Build history of the part. All positions in model axes, mm. A direction names the side the tool comes from. Give positions to 0.01 mm unless a question says otherwise; leave off trailing zeros. Order: outer loops, then holes, each group sorted by start corner. A loop starts at its lowest first (then second) coordinate and runs counter-clockwise, first axis right, second up. Notation, with made-up numbers: (2.5, 6.5) -> (56.5, 6.5) arc R31 cw to (56.5, 43.5) -> close; hole circle Ø2 at (27, 12). An arc over 180 degrees is marked (long way). Write item = value, one per line. Start each with the question number.
from build123d import *

# Parameters (mm, degrees)
SKETCH_1_W               = 74
SKETCH_1_H               = 52
EXTRUDE_1_DEPTH          = 2
CUT_EXTRUDE_2_DEPTH      = 10
SKETCH_3_W               = 2
SKETCH_3_H               = 8
EXTRUDE_3_DEPTH          = 7.5
FILLET_1_R               = 2
FILLET_1_OF_MIRROR_3_R   = 2
MIRROR_4_DEPTH           = 2
EXTRUDE_4_DEPTH          = 2
FILLET_3_R               = 1
FILLET_4_R               = 2
SKETCH_4_R               = 1.5
CUT_EXTRUDE_3_DEPTH      = 6
SKETCH_5_R               = 1
CUT_EXTRUDE_5_DEPTH      = 6
MIRROR_6_COPY_1_SKETCH_R = 1
MIRROR_6_COPY_1_DEPTH    = 6
SKETCH_6_R               = 1
CUT_EXTRUDE_6_DEPTH      = 10
MIRROR_9_COPY_1_SKETCH_R = 1
MIRROR_9_COPY_1_DEPTH    = 10
FILLET_5_R               = 1
CUT_EXTRUDE_7_DEPTH      = 10
MIRROR_12_COPY_1_DEPTH   = 10


# Read off the part's stored shape, not the designer's step: 镜向4
with BuildPart() as part:
    # 草图1 → 凸台-拉伸1 (new body)
    with BuildSketch(Plane(origin=(0, 0, 0), x_dir=(0, 0, -1), z_dir=(1, 0, 0))):
        Rectangle(SKETCH_1_W, SKETCH_1_H)
    extrude(amount=EXTRUDE_1_DEPTH)

    # 草图2 → 切除-拉伸2 (cut)
    with BuildSketch(Plane(origin=(2, 0, 0), x_dir=(0, 0, -1), z_dir=(1, 0, 0))):
        Polygon((-7, 0), (-31, 26), (-37, 26), (-37, -26), (-31, -26), align=None)
        Polygon((17, 26), (-17, 26), (0, 7.583333333), align=None)
        Polygon((31, 26), (7, 0), (31, -26), (37, -26), (37, 26), align=None)
        Polygon((17, -26), (0, -7.583333333), (-17, -26), align=None)
    extrude(amount=-CUT_EXTRUDE_2_DEPTH, mode=Mode.SUBTRACT)

    # 草图3 → 凸台-拉伸3 (add)
    with BuildSketch(Plane(origin=(0, 26, 0), x_dir=(1, 0, 0), z_dir=(0, 1, 0))):
        with Locations((1, -24)):
            Rectangle(SKETCH_3_W, SKETCH_3_H)
    extrude_3 = extrude(amount=EXTRUDE_3_DEPTH)

    # 圆角1
    fillet_1_edges = [part.edges().sort_by_distance(p)[0] for p in [
        (1, 33.5, 28),
        (1, 33.5, 20),
    ]]
    fillet(fillet_1_edges, radius=FILLET_1_R)

    # 镜向3: 凸台-拉伸3 across plane
    add(extrude_3.mirror(Plane.XY))

    # 圆角1 of 镜向3
    fillet_1_of_mirror_3_edges = [part.edges().sort_by_distance(p)[0] for p in [
        (1, 33.5, -28),
        (1, 33.5, -20),
    ]]
    fillet(fillet_1_of_mirror_3_edges, radius=FILLET_1_OF_MIRROR_3_R)

    # 镜向4 outline → 镜向4 (add)
    with BuildSketch(Plane.YZ):
        with BuildLine():
            Line((-26, 20), (-26, 28))
            Line((-26, 28), (-31.5, 28))
            ThreePointArc((-31.5, 28), (-32.914213562, 27.414213562), (-33.5, 26))
            Line((-33.5, 26), (-33.5, 22))
            ThreePointArc((-33.5, 22), (-32.914213562, 20.585786438), (-31.5, 20))
            Line((-31.5, 20), (-26, 20))
        make_face()
        with BuildLine():
            Line((-26, -20), (-31.5, -20))
            ThreePointArc((-31.5, -20), (-32.914213562, -20.585786438), (-33.5, -22))
            Line((-33.5, -22), (-33.5, -26))
            ThreePointArc((-33.5, -26), (-32.914213562, -27.414213562), (-31.5, -28))
            Line((-31.5, -28), (-26, -28))
            Line((-26, -28), (-26, -20))
        make_face()
    extrude(amount=MIRROR_4_DEPTH)

    # 草图7 → 凸台-拉伸4 (add)
    with BuildSketch(Plane(origin=(2, 0, 0), x_dir=(0, 0, -1), z_dir=(1, 0, 0))):
        Polygon((-28, 26), (-33, 26), (-33, 21.44166802), (-19, 13), align=None)
        Polygon((19, 13), (28, 26), (33, 26), (33, 21.44166802), align=None)
        Polygon((28, -26), (33, -26), (33, -21.44166802), (19, -13), align=None)
        Polygon((-19, -13), (-28, -26), (-33, -26), (-33, -21.44166802), align=None)
    extrude(amount=-EXTRUDE_4_DEPTH)

    # 圆角3
    fillet_3_edges = [part.edges().sort_by_distance(p)[0] for p in [
        (1, 26, 33),
        (1, 21.44166802, 33),
        (1, 26, -33),
        (1, 21.44166802, -33),
        (1, -26, -33),
        (1, -21.44166802, -33),
        (1, -26, 33),
        (1, -21.44166802, 33),
    ]]
    fillet(fillet_3_edges, radius=FILLET_3_R)

    # 圆角4
    fillet_4_edges = [part.edges().sort_by_distance(p)[0] for p in [
        (1, 0, -7),
        (1, 26, -17),
        (1, 7.583333333, 0),
        (1, 26, 17),
        (1, -7.583333333, 0),
        (1, -26, -17),
        (1, -26, 17),
        (1, 0, 7),
    ]]
    fillet(fillet_4_edges, radius=FILLET_4_R)

    # 草图4 → 切除-拉伸3 (cut)
    with BuildSketch(Plane(origin=(2, 0, 0), x_dir=(0, 0, -1), z_dir=(1, 0, 0))):
        with Locations((0, -4.5)):
            Circle(SKETCH_4_R)
        with Locations((-4.5, 0)):
            Circle(SKETCH_4_R)
        with Locations((0, 4.5)):
            Circle(SKETCH_4_R)
        with Locations((4.5, 0)):
            Circle(SKETCH_4_R)
    extrude(amount=-CUT_EXTRUDE_3_DEPTH, mode=Mode.SUBTRACT)

    # 草图5 → 切除-拉伸5 (cut)
    with BuildSketch(Plane(origin=(2, 0, 0), x_dir=(0, 0, -1), z_dir=(1, 0, 0))):
        with Locations((-24, 30.5)):
            Circle(SKETCH_5_R)
        with BuildLine():
            ThreePointArc((-23, 30.5), (-24, 29.5), (-25, 30.5))
            Line((-25, 30.5), (-25, 23.5))
            ThreePointArc((-25, 23.5), (-24, 24.5), (-23, 23.5))
            Line((-23, 23.5), (-23, 30.5))
        make_face()
        with Locations((-24, 23.5)):
            Circle(SKETCH_5_R)
    cut_extrude_5 = extrude(amount=-CUT_EXTRUDE_5_DEPTH, mode=Mode.SUBTRACT)

    # 镜向5: 切除-拉伸5 across plane
    add(cut_extrude_5.mirror(Plane.XY), mode=Mode.SUBTRACT)

    # 镜向6: 切除-拉伸5 across plane
    add(cut_extrude_5.mirror(Plane.ZX), mode=Mode.SUBTRACT)

    # 镜向6 copy 1 sketch → 镜向6 copy 1 (cut)
    with BuildSketch(Plane(origin=(2, 0, 0), x_dir=(0, 0, 1), z_dir=(1, 0, 0))):
        with Locations((-24, 30.5)):
            Circle(MIRROR_6_COPY_1_SKETCH_R)
        with BuildLine():
            ThreePointArc((-23, 30.5), (-24, 29.5), (-25, 30.5))
            Line((-25, 30.5), (-25, 23.5))
            ThreePointArc((-25, 23.5), (-24, 24.5), (-23, 23.5))
            Line((-23, 23.5), (-23, 30.5))
        make_face()
        with Locations((-24, 23.5)):
            Circle(MIRROR_6_COPY_1_SKETCH_R)
    extrude(amount=-MIRROR_6_COPY_1_DEPTH, mode=Mode.SUBTRACT)

    # 草图6 → 切除-拉伸6 (cut)
    with BuildSketch(Plane(origin=(2, 0, 0), x_dir=(0, 0, -1), z_dir=(1, 0, 0))):
        with Locations((-20, 26)):
            Circle(SKETCH_6_R)
        with Locations((-28, 26)):
            Circle(SKETCH_6_R)
    cut_extrude_6 = extrude(amount=-CUT_EXTRUDE_6_DEPTH, mode=Mode.SUBTRACT)

    # 镜向8: 切除-拉伸6 across plane
    add(cut_extrude_6.mirror(Plane.ZX), mode=Mode.SUBTRACT)

    # 镜向9: 切除-拉伸6 across plane
    add(cut_extrude_6.mirror(Plane.XY), mode=Mode.SUBTRACT)

    # 镜向9 copy 1 sketch → 镜向9 copy 1 (cut)
    with BuildSketch(Plane(origin=(2, 0, 0), x_dir=(0, 0, 1), z_dir=(1, 0, 0))):
        with Locations((-20, 26)):
            Circle(MIRROR_9_COPY_1_SKETCH_R)
        with Locations((-28, 26)):
            Circle(MIRROR_9_COPY_1_SKETCH_R)
    extrude(amount=-MIRROR_9_COPY_1_DEPTH, mode=Mode.SUBTRACT)

    # 圆角5
    fillet_5_edges = [part.edges().sort_by_distance(p)[0] for p in [
        (1, 27, 20),
        (1, 27, 28),
        (1, 26, 19),
        (1, 26, 29),
        (1, -27, 28),
        (1, -27, 20),
        (1, -26, 19),
        (1, -26, 29),
        (1, -27, -20),
        (1, -27, -28),
        (1, -26, -19),
        (1, -26, -29),
        (1, 27, -28),
        (1, 27, -20),
        (1, 26, -19),
        (1, 26, -29),
    ]]
    fillet(fillet_5_edges, radius=FILLET_5_R)

    # 草图8 → 切除-拉伸7 (cut)
    with BuildSketch(Plane(origin=(2, 0, 0), x_dir=(0, 0, -1), z_dir=(1, 0, 0))):
        with BuildLine():
            Line((-15.289196292, 19.511930318), (-6.669754344, 10.174201541))
            ThreePointArc((-6.669754344, 10.174201541), (-6.782801027, 7.348034446), (-9.608968122, 7.46108113))
            Line((-9.608968122, 7.46108113), (-18.22841007, 16.798809907))
            ThreePointArc((-18.22841007, 16.798809907), (-18.115363387, 19.624977002), (-15.289196292, 19.511930318))
        make_face()
    cut_extrude_7 = extrude(amount=-CUT_EXTRUDE_7_DEPTH, mode=Mode.SUBTRACT)

    # 镜向11: 切除-拉伸7 across plane
    add(cut_extrude_7.mirror(Plane.XY), mode=Mode.SUBTRACT)

    # 镜向12: 切除-拉伸7 across plane
    add(cut_extrude_7.mirror(Plane.ZX), mode=Mode.SUBTRACT)

    # 镜向12 copy 1 sketch → 镜向12 copy 1 (cut)
    with BuildSketch(Plane(origin=(2, 0, 0), x_dir=(0, 0, 1), z_dir=(1, 0, 0))):
        with BuildLine():
            Line((-15.289196292, 19.511930318), (-6.669754344, 10.174201541))
            ThreePointArc((-6.669754344, 10.174201541), (-6.782801027, 7.348034446), (-9.608968122, 7.46108113))
            Line((-9.608968122, 7.46108113), (-18.22841007, 16.798809907))
            ThreePointArc((-18.22841007, 16.798809907), (-18.115363387, 19.624977002), (-15.289196292, 19.511930318))
        make_face()
    extrude(amount=-MIRROR_12_COPY_1_DEPTH, mode=Mode.SUBTRACT)


solid = part.part
(1) Cut at D-D, the plane x = 0.7. Give the number of separate pieces and of enclosed holes in the cut face, plus the area to 3 significant figures.
(2) Mould opens along Z. For faces 5 (the face through (1.01, -17.13, -25.85)), 6 (the face through (1.01, 17.15, -8.83)), 7 (the face through (1.01, -7.26, 13.7)) say: released by +Z, released by -Z, zero draft, split by the parting line, or undercut.
(3) 3-axis set-ups, long thin cutter, end or side, ignore diameter. For faces 1 (the face through (0.986, 25.837, 17.084)), 2 (the face through (1, -31.5, 24)), 3 (the face through (0.986, -25.837, 17.084)), 4 (the face through (1, -30, 28)): which of +Z, -Z, +X, -X, +Y, -Y reach the whole face in a straight line?
(4) Flat gauge pins, fed straight in: P1, Ø0.6, axis at x = 1.5, y = -27.5, coming from the +Z side; P2, Ø1.6, axis at y = 26, z = 28, coming from the -X side; P3, Ø1, axis at y = -14.5, z = -9, coming from the -X side. Where does each tip first touch, or does it go through?
(5) Wall check: line 1 (Z direction, x = 1.2, y = -28); line 2 (Y direction, x = 1.5, z = 0); line 3 (Z direction, x = 1.1, y = 27). Give the ranges that are in metal, low to high. Write a range as [from, to].
(6) Cut at C-C, the plane z = -14.5. Give the cut face in (x, y) (3 decimals).
(7) Cut at A-A, the plane z = 0. Give the cut face in (x, y).
(8) Cut at B-B, the plane y = 15.5. Give the cut face in (x, z), plus the area to 3 significant figures.
Results:
q1.separate_pieces = 1
q1.enclosed_holes = 12
q1.area = 1,390 mm2
q2.face_5 = released by -Z
q2.face_6 = undercut
q2.face_7 = released by +Z
q3.face_1 = +X, -X, +Y
q3.face_2 = +X, -X
q3.face_3 = +X, -X, -Y
q3.face_4 = +Z, +X, -X, -Y
q4.P1 = 28
q4.P2 = through
q4.P3 = 0
q5.line_1 = [-28, -25], [-23, -20], [20, 23], [25, 28]
q5.line_2 = [-8.53, -6], [-3, 3], [6, 8.53]
q5.line_3 = [-27.68, -25], [-23, -20.32], [20.32, 23], [25, 27.68]
q6.outline = (0, -23.292) -> (2, -23.292) -> (2, -18.657) -> (0, -18.657) -> close; (0, -12.76) -> (2, -12.76) -> (2, -8.125) -> (0, -8.125) -> close; (0, 8.125) -> (2, 8.125) -> (2, 12.76) -> (0, 12.76) -> close; (0, 18.657) -> (2, 18.657) -> (2, 23.292) -> (0, 23.292) -> close
q7.outline = (0, -8.53) -> (2, -8.53) -> (2, -6) -> (0, -6) -> close; (0, -3) -> (2, -3) -> (2, 3) -> (0, 3) -> close; (0, 6) -> (2, 6) -> (2, 8.53) -> (0, 8.53) -> close
q8.outline = (0, -23.15) -> (2, -23.15) -> (2, -17.03) -> (0, -17.03) -> close; (0, -11.59) -> (2, -11.59) -> (2, -7.31) -> (0, -7.31) -> close; (0, 7.31) -> (2, 7.31) -> (2, 11.59) -> (0, 11.59) -> close; (0, 17.03) -> (2, 17.03) -> (2, 23.15) -> (0, 23.15) -> close
q8.area = 41.6 mm2
